CAD build for the part. Positions are in the model's coordinates, mm. A direction names the side the tool comes from. Coordinates: 2 decimals unless noted, no trailing zeros. Write each loop counter-clockwise with the first axis right and the second up, starting at its lowest first coordinate (ties: lowest second). Pieces come first, ordered by that corner, then holes. Notation, with made-up numbers: (-3, 44) -> (11, 44) arc R25 cw to (11, 61) -> close; hole circle Ø8 at (74, 1). An arc over 180 degrees is marked (long way). Answer as CSV lines item,"result". Start each with the question number.
```python
from build123d import *

# Parameters (mm, degrees)
ESQUISSE1_W                   = 175
ESQUISSE1_H                   = 175
BOSS_EXTRU_1_DEPTH            = 4.500081728
BOSS_EXTRU_4_DEPTH            = 46
ESQUISSE12_W                  = 4
ESQUISSE12_H                  = 171
BOSS_EXTRU_5_DEPTH            = 15
ESQUISSE13_R                  = 2.5
ENL_V_MAT_EXTRU_1_DEPTH       = 15
ESQUISSE15_R                  = 2.5
ENL_V_MAT_EXTRU_2_DEPTH       = 253.587130026
ESQUISSE18_W                  = 10
ESQUISSE18_H                  = 155
ENL_V_MAT_EXTRU_3_DEPTH       = 15
ESQUISSE19_R                  = 1.625
ENL_V_MAT_EXTRU_4_DEPTH       = 15
CONG_4_R                      = 2
CONG_5_R                      = 2
CONG_6_R                      = 2
ESQUISSE22_R                  = 2.5
ENL_V_MAT_EXTRU_5_DEPTH       = 10
ESQUISSE27_W                  = 49.077912464
ESQUISSE27_H                  = 68.885759281
ESQUISSE27_W_2                = 65.156972179
ESQUISSE27_H_2                = 37.514528632
ESQUISSE27_W_3                = 33.342624299
ESQUISSE27_H_3                = 29.898225407
ESQUISSE27_W_4                = 70
ESQUISSE27_H_4                = 10
ESQUISSE27_W_5                = 55.665773392
ESQUISSE27_H_5                = 20
ENL_V_MAT_EXTRU_8_DEPTH       = 7.5
BOSS_EXTRU_8_REACH            = 253.206
ESQUISSE28_W                  = 6
ESQUISSE28_H                  = 3
ESQUISSE29_R                  = 2
ENL_V_MAT_EXTRU_9_DEPTH       = 3
ENL_V_MAT_EXTRU_10_DEPTH      = 199
ENL_V_MAT_EXTRU_10_DEPTH_BACK = 10
ESQUISSE30_R                  = 3
ESQUISSE30_R_2                = 2


with BuildPart() as part:
    # Esquisse1 → Boss.-Extru.1 (new body)
    with BuildSketch(Plane.XY):
        with Locations((87.5, 87.5)):
            Rectangle(ESQUISSE1_W, ESQUISSE1_H)
    extrude(amount=BOSS_EXTRU_1_DEPTH)

    # Esquisse9 → Boss.-Extru.4 (add)
    with BuildSketch(Plane.XY.offset(4.500081728)):
        Polygon((0, 2), (0, 0), (172, 0), (175, 0), (175, 4), (175, 146), (175, 175), (173, 175), (0, 175), (0, 173), (173, 173), (173, 2), align=None)
    extrude(amount=BOSS_EXTRU_4_DEPTH)

    # Esquisse12 → Boss.-Extru.5 (add)
    with BuildSketch(Plane.ZY.offset(-173)):
        with Locations((48.500081728, 87.5)):
            Rectangle(ESQUISSE12_W, ESQUISSE12_H)
    extrude(amount=BOSS_EXTRU_5_DEPTH)

    # Esquisse13 → Enlèv. mat.-Extru.1 (cut)
    with BuildSketch(Plane.XY.offset(50.500081728)):
        with Locations((162.695433775, 82.004217199)):
            Circle(ESQUISSE13_R)
        with Locations((163, 93)):
            Circle(ESQUISSE13_R)
    extrude(amount=-ENL_V_MAT_EXTRU_1_DEPTH, mode=Mode.SUBTRACT)

    # Esquisse15 → Enlèv. mat.-Extru.2 (cut, through all)
    with BuildSketch(Plane.XZ):
        with Locations(Location((10, 25.500081728, 0), (0, 0, 270))):
            Circle(ESQUISSE15_R)
    extrude(amount=-ENL_V_MAT_EXTRU_2_DEPTH, mode=Mode.SUBTRACT)

    # Esquisse18 → Enlèv. mat.-Extru.3 (cut)
    with BuildSketch(Plane(origin=(0, 0, 0), x_dir=(-1, 0, 0), z_dir=(0, 0, -1))):
        with Locations((-160, 87.5)):
            Rectangle(ESQUISSE18_W, ESQUISSE18_H)
    extrude(amount=-ENL_V_MAT_EXTRU_3_DEPTH, mode=Mode.SUBTRACT)

    # Esquisse19 → Enlèv. mat.-Extru.4 (cut)
    with BuildSketch(Plane(origin=(0, 0, 0), x_dir=(-1, 0, 0), z_dir=(0, 0, -1))):
        with Locations((-92.63, 150)):
            Circle(ESQUISSE19_R)
        with Locations((-10, 150)):
            Circle(ESQUISSE19_R)
        with Locations((-10, 101.66)):
            Circle(ESQUISSE19_R)
    extrude(amount=-ENL_V_MAT_EXTRU_4_DEPTH, mode=Mode.SUBTRACT)

    # Congé4
    cong_4_edges = [part.edges().sort_by_distance(p)[0] for p in [
        (173, 87.5, 46.500081728),
    ]]
    fillet(cong_4_edges, radius=CONG_4_R)

    # Congé5
    cong_5_edges = [part.edges().sort_by_distance(p)[0] for p in [
        (175, 87.5, 50.500081728),
    ]]
    fillet(cong_5_edges, radius=CONG_5_R)

    # Congé6
    cong_6_edges = [part.edges().sort_by_distance(p)[0] for p in [
        (175, 87.5, 0),
    ]]
    fillet(cong_6_edges, radius=CONG_6_R)

    # Esquisse22 → Enlèv. mat.-Extru.5 (cut)
    with BuildSketch(Plane(origin=(0, 0, 0), x_dir=(-1, 0, 0), z_dir=(0, 0, -1))):
        with Locations((-15, 15)):
            Circle(ESQUISSE22_R)
        with Locations((-65, 15)):
            Circle(ESQUISSE22_R)
        with Locations((-65, 60)):
            Circle(ESQUISSE22_R)
        with Locations((-15, 60)):
            Circle(ESQUISSE22_R)
    extrude(amount=-ENL_V_MAT_EXTRU_5_DEPTH, mode=Mode.SUBTRACT)

    # Esquisse27 → Enlèv. mat.-Extru.8 (cut)
    with BuildSketch(Plane(origin=(0, 0, 0), x_dir=(-1, 0, 0), z_dir=(0, 0, -1))):
        with Locations((-130.461043768, 130.55712036)):
            Rectangle(ESQUISSE27_W, ESQUISSE27_H)
        with Locations((-47.57848609, 125.547945711)):
            Rectangle(ESQUISSE27_W_2, ESQUISSE27_H_2)
        with Locations((-42.34290333, 39.239653333)):
            Rectangle(ESQUISSE27_W_3, ESQUISSE27_H_3)
        with Locations((-50, 164.354328762)):
            Rectangle(ESQUISSE27_W_4, ESQUISSE27_H_4)
        with Locations((-42.832886696, 80.328302815)):
            Rectangle(ESQUISSE27_W_5, ESQUISSE27_H_5)
    extrude(amount=-ENL_V_MAT_EXTRU_8_DEPTH, mode=Mode.SUBTRACT)

    # Esquisse28 → Boss.-Extru.8 (add, up to next)
    with BuildSketch(Plane(origin=(0, 2, 0), x_dir=(1, 0, 0), z_dir=(0, 1, 0)), mode=Mode.PRIVATE) as boss_extru_8_sk1:
        with Locations((35.927740349, -49.000081728)):
            Rectangle(ESQUISSE28_W, ESQUISSE28_H)
    boss_extru_8_tool1 = extrude(boss_extru_8_sk1.sketch, amount=BOSS_EXTRU_8_REACH, mode=Mode.PRIVATE) - part.part
    # Esquisse28 → Boss.-Extru.8 (add, up to next)
    with BuildSketch(Plane(origin=(0, 2, 0), x_dir=(1, 0, 0), z_dir=(0, 1, 0)), mode=Mode.PRIVATE) as boss_extru_8_sk2:
        with Locations((56.927740349, -49.000081728)):
            Rectangle(ESQUISSE28_W, ESQUISSE28_H)
    boss_extru_8_tool2 = extrude(boss_extru_8_sk2.sketch, amount=BOSS_EXTRU_8_REACH, mode=Mode.PRIVATE) - part.part
    add(boss_extru_8_tool1.solids().sort_by_distance((35.92774, 2, 49.000082))[0])
    add(boss_extru_8_tool2.solids().sort_by_distance((56.92774, 2, 49.000082))[0])

    # Esquisse29 → Enlèv. mat.-Extru.9 (cut)
    with BuildSketch(Plane.XY.offset(50.500081728)):
        with Locations((56.927740349, 74.5)):
            Circle(ESQUISSE29_R)
        with Locations((35.927740349, 74.5)):
            Circle(ESQUISSE29_R)
        with Locations((56.927740349, 52.5)):
            Circle(ESQUISSE29_R)
        with Locations((35.927740349, 52.5)):
            Circle(ESQUISSE29_R)
        with Locations((56.927740349, 100.5)):
            Circle(ESQUISSE29_R)
        with Locations((35.927740349, 100.5)):
            Circle(ESQUISSE29_R)
        with Locations((35.927740349, 122.5)):
            Circle(ESQUISSE29_R)
        with Locations((56.927740349, 122.5)):
            Circle(ESQUISSE29_R)
    extrude(amount=-ENL_V_MAT_EXTRU_9_DEPTH, mode=Mode.SUBTRACT)

    # Esquisse30 → Enlèv. mat.-Extru.10 (cut, two sides: drawn at the far end of the back side and taken through both)
    with BuildSketch(Plane(origin=(0, 2, 0), x_dir=(1, 0, 0), z_dir=(0, 1, 0)).offset(-ENL_V_MAT_EXTRU_10_DEPTH_BACK)):
        with Locations((61, -30.500081728)):
            Circle(ESQUISSE30_R)
        with Locations((82.2, -39.000081728)):
            Circle(ESQUISSE30_R_2)
        with Locations((82.2, -22.000081728)):
            Circle(ESQUISSE30_R_2)
    extrude(amount=ENL_V_MAT_EXTRU_10_DEPTH + ENL_V_MAT_EXTRU_10_DEPTH_BACK, mode=Mode.SUBTRACT)


solid = part.part
```
1. Flat gauge pins, fed straight in: P1, Ø8, axis at y = 77.5, z = 19, coming from the -X side; P2, Ø4.5, axis at x = 10, z = 25.5, coming from the -Y side; P3, Ø10, axis at x = 110.5, y = 100, coming from the +Z side. Where does each tip first touch, or does it go through?
2. Cut at B-B (x = 130.5). Give the cut face in (y, z).
3. Cut at D-D (x = 99.5). Give the cut face in (y, z), then the cut area to 3 significant figures.
4. Mould opens along Y. For faces 1 (the face through (85, 70, 4.5)), 2 (the face through (0, 88, 1)) say: pulls with the +Y half, pulls with the -Y half, needs draft (parallel to the pull), parting line crosses it, or undercut.
5. Tool access for faces 3 (the face through (131, 96.114, 2)), 4 (the face through (80.202, 0.986, 21.912)), 5 (the face through (160, 10, 2)), 6 (the face through (165, 86, 46.5)), 7 (the face through (56.667, 102.483, 49.021)): list every direction of +Z, -Z, +X, -X, +Y, -Y with a clear straight run to the whole face (end or side of a thin tool).
6. Cut at C-C (y = 20.5). Give the cut face in (x, z).
7. Cut at A-A (y = 38.5). Give the cut face in (x, z).
8. Wall check: line 1 (Y direction, x = 119, z = 27); line 2 (X direction, y = 23.5, z = 3); line 3 (X direction, y = 100, z = 49). Give the ranges that are in metal, low to high.
Geometry check:
1,P1,"x = 173"
1,P2,"through"
1,P3,"z = 4.5"
2,outline,"(0, 0) -> (96.11, 0) -> (96.11, 4.5) -> (2, 4.5) -> (2, 50.5) -> (0, 50.5) -> close; (165, 0) -> (175, 0) -> (175, 50.5) -> (173, 50.5) -> (173, 4.5) -> (165, 4.5) -> close"
3,outline,"(0, 0) -> (175, 0) -> (175, 50.5) -> (173, 50.5) -> (173, 4.5) -> (2, 4.5) -> (2, 50.5) -> (0, 50.5) -> close"
3,area,"972 mm²"
4,face 1,"undercut"
4,face 2,"needs draft"
5,face 3,"+Z, -Z"
5,face 4,"+Y, -Y"
5,face 5,"-Z"
5,face 6,"-X"
5,face 7,"+Z"
6,outline,"(0, 0) -> (155, 0) -> (155, 4.5) -> (0, 4.5) -> close; (32.93, 47.5) -> (38.93, 47.5) -> (38.93, 50.5) -> (32.93, 50.5) -> close; (53.93, 47.5) -> (59.93, 47.5) -> (59.93, 50.5) -> (53.93, 50.5) -> close; (158, 46.5) -> (171, 46.5) arc R2 cw to (173, 44.5) -> (173, 4.5) -> (165, 4.5) -> (165, 0) -> (173, 0) arc R2 ccw to (175, 2) -> (175, 48.5) arc R2 ccw to (173, 50.5) -> (158, 50.5) -> close"
7,outline,"(0, 0) -> (25.67, 0) -> (25.67, 4.5) -> (0, 4.5) -> close; (32.93, 47.5) -> (38.93, 47.5) -> (38.93, 50.5) -> (32.93, 50.5) -> close; (53.93, 47.5) -> (59.93, 47.5) -> (59.93, 50.5) -> (53.93, 50.5) -> close; (59.01, 0) -> (155, 0) -> (155, 4.5) -> (59.01, 4.5) -> close; (158, 46.5) -> (171, 46.5) arc R2 cw to (173, 44.5) -> (173, 4.5) -> (165, 4.5) -> (165, 0) -> (173, 0) arc R2 ccw to (175, 2) -> (175, 48.5) arc R2 ccw to (173, 50.5) -> (158, 50.5) -> close"
8,line 1,"0 to 2, 173 to 175"
8,line 2,"0 to 155, 165 to 175"
8,line 3,"32.93 to 33.99, 37.86 to 38.93, 53.93 to 54.99, 58.86 to 59.93, 158 to 174.94"
